Could you check a few things on this model? Use its own coordinates, in mm. A direction names the side the tool comes from. Coordinates: 2 decimals unless noted, no trailing zeros. Order: outer loops, then holes, each group sorted by start corner. A loop starts at its lowest first (then second) coordinate and runs counter-clockwise, first axis right, second up. Notation, with made-up numbers: (28, 8.5) -> (46, 8.5) arc R24 ccw to (46, 31.5) -> close; hole circle Ø4 at (-7, 83.5). An arc over 180 degrees is marked (long way). Put each result on its own line as item: value. Start each with the question number.
Q1. If we section it at A-A (x = 0): Please give me the cut outline in (y, z) (3 decimals), and give its area (4 significant figures).
Q2. We'd pull the mould along Y, two halves only. Please class faces 1 (the face through (4, 9, 5)), 2 (the face through (-6.37, 0.74, 4.88)), 3 (the face through (2, 0, -2)): +Y half, -Y half, draft (parallel to the pull), parting line (faces both ways), or undercut.
Q3. Please list where these lines run through material, in increasing order: line 1 along Z through (x, y) = (0, 5); line 2 along Y through (x, z) = (0, -6.5).
Q4. Will these pins go through, and if not, where does the flat tip stop? pin 1 (1.5 mm diameter, centred on y = 1.5, z = 2, fed in from +X); pin 2 (1 mm diameter, centred on y = 6, z = 3.5, fed in from +X); pin 3 (4 mm diameter, centred on x = -1.5, y = 4, fed in from +Z).
Q5. If we section it at B-B (z = 0): Please give me the cut outline in (x, y) (3 decimals), and give its area (4 significant figures).
Q6. If we section it at C-C (y = 2.5): Please give me the cut outline in (x, z).
Q7. For faces 4 (the face through (4, 1.5, 5)), 5 (the face through (2, 10.5, -2)), which set-ups out of +Z, -Z, +X, -X, +Y, -Y let a thin tool reach every point of the face, with its end or its side?
Q8. If we section it at D-D (x = -2.75): Please give me the cut outline in (y, z), and give its area (3 significant figures).
from build123d import *

# Parameters (mm, degrees)
SKETCH1_R           = 8.025
BOSS_EXTRUDE1_DEPTH = 1.5
SKETCH2_R           = 6.2
BOSS_EXTRUDE2_DEPTH = 7.5
SKETCH3_R           = 8.025
BOSS_EXTRUDE3_DEPTH = 1.5
SKETCH4_R           = 2.5
CUT_EXTRUDE1_DEPTH  = 11.5


with BuildPart() as part:
    # Sketch1 → Boss-Extrude1 (new body)
    with BuildSketch(Plane(origin=(0, 0, 0), x_dir=(1, 0, 0), z_dir=(0, 1, 0))):
        Circle(SKETCH1_R)
    extrude(amount=BOSS_EXTRUDE1_DEPTH)

    # Sketch2 → Boss-Extrude2 (add)
    with BuildSketch(Plane(origin=(0, 1.5, 0), x_dir=(1, 0, 0), z_dir=(0, 1, 0))):
        Circle(SKETCH2_R)
    extrude(amount=BOSS_EXTRUDE2_DEPTH)

    # Sketch3 → Boss-Extrude3 (add)
    with BuildSketch(Plane(origin=(0, 9, 0), x_dir=(1, 0, 0), z_dir=(0, 1, 0))):
        Circle(SKETCH3_R)
    extrude(amount=BOSS_EXTRUDE3_DEPTH)

    # Sketch4 → Cut-Extrude1 (cut, through all)
    with BuildSketch(Plane(origin=(0, 10.5, 0), x_dir=(1, 0, 0), z_dir=(0, 1, 0))):
        Circle(SKETCH4_R)
    extrude(amount=-CUT_EXTRUDE1_DEPTH, mode=Mode.SUBTRACT)


solid = part.part
The answers:
1. outline: (0, -8.025) -> (1.5, -8.025) -> (1.5, -6.2) -> (9, -6.2) -> (9, -8.025) -> (10.5, -8.025) -> (10.5, -2.5) -> (0, -2.5) -> close; (0, 2.5) -> (10.5, 2.5) -> (10.5, 8.025) -> (9, 8.025) -> (9, 6.2) -> (1.5, 6.2) -> (1.5, 8.025) -> (0, 8.025) -> close
1. area: 88.65 mm^2
2. face 1: undercut
2. face 2: draft
2. face 3: -Y half
3. line 1: -6.2 to -2.5, 2.5 to 6.2
3. line 2: 0 to 1.5, 9 to 10.5
4. pin 1: x = 7.93
4. pin 2: x = 5.43
4. pin 3: z = 6.2
5. outline: (-8.025, 0) -> (-2.5, 0) -> (-2.5, 10.5) -> (-8.025, 10.5) -> (-8.025, 9) -> (-6.2, 9) -> (-6.2, 1.5) -> (-8.025, 1.5) -> close; (2.5, 0) -> (8.025, 0) -> (8.025, 1.5) -> (6.2, 1.5) -> (6.2, 9) -> (8.025, 9) -> (8.025, 10.5) -> (2.5, 10.5) -> close
5. area: 88.65 mm^2
6. outline: circle Ø12.4 at (0, 0); hole circle Ø5 at (0, 0)
7. face 4: none
7. face 5: +Z, -Z, +X, -X, +Y
8. outline: (0, -7.54) -> (1.5, -7.54) -> (1.5, -5.56) -> (9, -5.56) -> (9, -7.54) -> (10.5, -7.54) -> (10.5, 7.54) -> (9, 7.54) -> (9, 5.56) -> (1.5, 5.56) -> (1.5, 7.54) -> (0, 7.54) -> close
8. area: 129 mm^2
